from build123d import *

# Parameters (mm, degrees)
SKETCH1_R           = 2.25
BOSS_EXTRUDE1_DEPTH = 10
SKETCH2_R           = 2.25
CUT_EXTRUDE1_DEPTH  = 11


with BuildPart() as part:
    # Sketch1 → Boss-Extrude1 (new body)
    with BuildSketch(Plane.XY):
        Polygon((-60, -5), (60, -5), (60, 5), (25, 105), (-25, 105), (-60, 5), align=None)
        with Locations((27.5, 0)):
            Circle(SKETCH1_R, mode=Mode.SUBTRACT)
        with Locations((12.5, 0)):
            Circle(SKETCH1_R, mode=Mode.SUBTRACT)
        with Locations((-12.5, 0)):
            Circle(SKETCH1_R, mode=Mode.SUBTRACT)
        with Locations((-27.5, 0)):
            Circle(SKETCH1_R, mode=Mode.SUBTRACT)
    extrude(amount=BOSS_EXTRUDE1_DEPTH)

    # Sketch2 → Cut-Extrude1 (cut, through all)
    with BuildSketch(Plane.XY.offset(10)):
        with Locations((-21.75, 80)):
            Circle(SKETCH2_R)
        with Locations((21.75, 80)):
            Circle(SKETCH2_R)
        with Locations((21.75, 100)):
            Circle(SKETCH2_R)
        with Locations((-21.75, 100)):
            Circle(SKETCH2_R)
    extrude(amount=-CUT_EXTRUDE1_DEPTH, mode=Mode.SUBTRACT)


solid = part.part
Part model, mm, in its own coordinate system. Coordinates: 2 decimals unless noted, no trailing zeros. Order: outer loops, then holes, each group sorted by start corner. A loop starts at its lowest first (then second) coordinate and runs counter-clockwise, first axis right, second up. Notation, with made-up numbers: (-10, 5) - (20, 5) arc R12 cw to (20, 22) - close; hole circle Ø4 at (3.5, 34). An arc over 180 degrees is marked (long way). Use CSV: the item, a comma, the result in double quotes.
Item 1: Saw through at A-A on y = 100. Give the cut face in (x, z), and give its area (3 significant figures).
Solved:
outline,"(-26.75, 0) - (-24, 0) - (-24, 10) - (-26.75, 10) - close; (-19.5, 0) - (19.5, 0) - (19.5, 10) - (-19.5, 10) - close; (24, 0) - (26.75, 0) - (26.75, 10) - (24, 10) - close"
area,"445 mm²"
Item 2: Probe probe 1 along Y at (x, z) = (-12.5, 7.25); probe 2 along Y at (x, z) = (22, 5.75); probe 3 along X at (y, z) = (59.5, 3.5) (3 decimals). List the from-to ranges inside material, lowest first.
Solved:
probe 1,"y = -5 to -2.25, 2.25 to 105"
probe 2,"y = -5 to 77.76, 82.24 to 97.76, 102.24 to 105"
probe 3,"x = -40.925 to 40.925"
Item 3: Mould opens along Y. For faces 1 (the face through (-1, 39, 0)), 2 (the face through (29.646, 0.676, 4.93)), 3 (the face through (-1, -5, 5)) say: +Y half, -Y half, draft (parallel to the pull), parting line (faces both ways), or undercut.
Solved:
face 1,"draft"
face 2,"undercut"
face 3,"-Y half"
Item 4: Drop flat-ended pins along their axis: P1, Ø1.5, axis at y = 22, z = 5.5, coming from the -X side; P2, Ø7, axis at x = 12.5, y = 0, coming from the -Z side; P3, Ø4, axis at y = 71.5, z = 5.5, coming from the -X side (3 decimals); P4, Ø2, axis at y = 17, z = 4.5, coming from the -X side. Give the stop position or say it passes through.
Solved:
P1,"stops at x = -54.31"
P2,"stops at z = 0"
P3,"stops at x = -37.425"
P4,"stops at x = -56.15"
Item 5: Saw through at C-C on x = 12.5. Give the cut face in (y, z).
Solved:
outline,"(-5, 0) - (-2.25, 0) - (-2.25, 10) - (-5, 10) - close; (2.25, 0) - (105, 0) - (105, 10) - (2.25, 10) - close"
Item 6: Saw through at D-D on z = 2.25. Give the number of separate pieces and of enclosed holes in the cut face, and give its area (3 significant figures).
Solved:
separate pieces,"1"
enclosed holes,"8"
area,"9,570 mm²"
Item 7: Saw through at B-B on x = -21.75. Give the cut face in (y, z), and give its area (3 significant figures).
Solved:
outline,"(-5, 0) - (77.75, 0) - (77.75, 10) - (-5, 10) - close; (82.25, 0) - (97.75, 0) - (97.75, 10) - (82.25, 10) - close; (102.25, 0) - (105, 0) - (105, 10) - (102.25, 10) - close"
area,"1,010 mm²"
